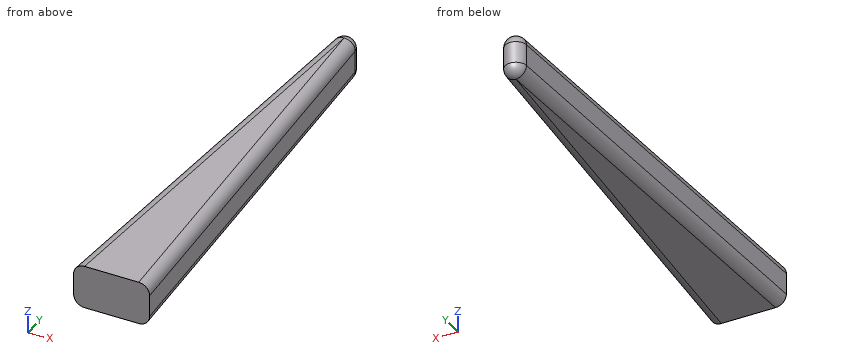
from build123d import *

# Parameters (mm, degrees)
F1_DEPTH = 4
F2_R     = 1


with BuildPart() as f1:
    # F0 (on Top) → F1 (new body)
    with BuildSketch(Plane.XY):
        with BuildLine():
            Line((-1, 40), (-3.5, 0))
            Line((-3.5, 0), (3.5, 0))
            Line((3.5, 0), (1, 40))
            ThreePointArc((1, 40), (0, 40.939451), (-1, 40))
        make_face()
    extrude(amount=F1_DEPTH)

    # F2
    f2_edges = [f1.edges().sort_by_distance(p)[0] for p in [
        (-2.25, 20, 4),
        (-2.25, 20, 0),
        (2.25, 20, 4),
        (2.25, 20, 0),
    ]]
    fillet(f2_edges, radius=F2_R)


solid = f1.part
Read the model definition and answer for the solid it produces. Units are mm, in the model's axes. Round coordinates to 2 decimals unless told otherwise and drop trailing zeros. Write each loop counter-clockwise with the first axis right and the second up, starting at its lowest first coordinate (ties: lowest second). Pieces come first, ordered by that corner, then holes.
1. Given pin 1 Ø1 at (y, z) = (20, 2) entering from -X; pin 2 Ø2 at (y, z) = (11.5, 1.5) entering from -X, each flat-ended and moving along its own axis, determine where each tip first touches the part or whether it passes through.
2. Straight lines are drawn through the part: L1, parallel to X at y = 12.5, z = 0.45; L2, parallel to X at y = 25, z = 1.75; L3, parallel to Y at x = 0.5, z = 0.75. For each, find the intervals that lie inside material, in ascending order.
3. The part is cut by section A-A, the plane z = 2.45. Determine the outline of the cut face in (x, y).
Values:
1. pin 1: stops at x = -2.28
1. pin 2: stops at x = -2.84
2. L1: x = -2.55 to 2.55
2. L2: x = -1.94 to 1.94
2. L3: y = 0 to 40.77
3. outline: (-3.5, 0) - (3.5, 0) - (1, 40) arc R1 ccw to (-1, 40) - close
